Input: part model. Units: mm. Frame: model coordinates. A direction names the side the tool comes from. Give positions to 0.01 mm unless a question says otherwise; leave off trailing zeros. Loops run counter-clockwise (first coordinate to the right, second up) from the corner with the lowest first, then second, coordinate; pieces in that order, holes last. Notation, with made-up numbers: (2.25, -33.75) - (17.25, -33.75) arc R17 ccw to (17.25, -14.75) - close; hole circle Ø10 at (69.5, 54). An arc over 180 degrees is marked (long way). Answer as a JSON object with one key per item and string values. Group by question number.
(1) Pin query (flat end, axial travel): P1, Ø10, axis at y = 1.5, z = 12, coming from the -X side; P2, Ø2, axis at y = 26, z = 8, coming from the +X side; P3, Ø3, axis at x = 11, y = 24.5, coming from the -Z side. Return the tip coordinate at first contact, or that it passes through.
(2) Section query B-B (z = 11.5). Return loops of the section in (x, y), plus the area to 3 significant figures.
(3) Mould query, pull axis X, two halves, no side actions, for faces 4 (the flat face through (3.127, -26.5, 11.3)), 5 (the flat face through (16, 0, 11)), 6 (the flat face through (6, -17.5, 11)). Classes: +X half, -X half, draft (parallel to the pull), parting line (faces both ways), or undercut.
(4) Section query A-A (x = 8.75). Return loops of the section in (y, z).
(5) Section query C-C (y = -23.4). Return loops of the section in (x, z), plus the area to 3 significant figures.
(6) Access query for faces 1 (the flat face through (13, 0, 11)), 2 (the flat face through (9, -23, 14.75)), 3 (the flat face through (8, 24, 14.75)). Directions: +Z, -Z, +X, -X, +Y, -Y. A direction counts if a zero-diameter tool reaches every point of the face in a straight line with its end or side. Return the directions, or none.
(7) Section query D-D (x = 12). Return loops of the section in (y, z), plus the area to 3 significant figures.
(8) Material intervals for L1, parallel to Y at x = 6.5, z = 3.75; L2, parallel to Z at x = 1.8, y = -24.25; L3, parallel to Y at x = 12.75, z = 15, sorted ascending.
```python
from build123d import *

# Parameters (mm, degrees)
BOSS_EXTRUDE1_DEPTH = 23
SKETCH2_R           = 1.7
CUT_EXTRUDE1_DEPTH  = 39.81958977
CUT_EXTRUDE5_START  = 23
SKETCH2_8_R         = 3.25
SKETCH2_8_R_2       = 1.7
CUT_EXTRUDE5_DEPTH  = 23
MIRROR5_START       = 14.75
MIRROR5_OUTLINE_W   = 3.127139018
MIRROR5_OUTLINE_H   = 0.5
MIRROR5_DEPTH       = 8.25
MIRROR5_2_OUTLINE_W = 3.127139018
MIRROR5_2_OUTLINE_H = 0.5
MIRROR5_2_DEPTH     = 14.75
MIRROR5_3_OUTLINE_W = 13
MIRROR5_3_OUTLINE_H = 0.5
MIRROR5_3_DEPTH     = 23
MIRROR5_4_OUTLINE_R = 1.7
MIRROR5_4_DEPTH     = 3.127139018
MIRROR5_5_OUTLINE_R = 1.7
MIRROR5_5_DEPTH     = 3.127139018
SKETCH5_R           = 1.7
CUT_EXTRUDE6_DEPTH  = 41.323690307
CUT_EXTRUDE7_DEPTH  = 23


with BuildPart() as part:
    # Sketch1 → Boss-Extrude1 (new body)
    with BuildSketch(Plane.XY):
        with BuildLine():
            Line((13, 18), (13, -18))
            Line((13, -18), (0, -18))
            Line((0, -18), (0, -28.5))
            Line((0, -28.5), (3.127139018, -28.5))
            Line((3.127139018, -28.5), (3.127139018, -21))
            Line((3.127139018, -21), (16, -21))
            Line((16, -21), (16, 21))
            ThreePointArc((16, 21), (9.563569509, 27.436430491), (3.127139018, 21))
            Line((3.127139018, 21), (3.127139018, 28.5))
            Line((3.127139018, 28.5), (0, 28.5))
            Line((0, 28.5), (0, 18))
            Line((0, 18), (13, 18))
        make_face()
    extrude(amount=BOSS_EXTRUDE1_DEPTH)

    # Sketch2 → Cut-Extrude1 (cut, symmetric)
    with BuildSketch(Plane(origin=(3.127139018, 0, 0), x_dir=(0, 0, -1), z_dir=(1, 0, 0))):
        with Locations((-11.5, 24.75)):
            Circle(SKETCH2_R)
    extrude(amount=CUT_EXTRUDE1_DEPTH, both=True, mode=Mode.SUBTRACT)

    # Sketch2_8 → Cut-Extrude5 (cut)
    # profile 1 of 4: a face of its own
    with BuildSketch(Plane(origin=(3.127139018, 0, 0), x_dir=(0, 0, -1), z_dir=(1, 0, 0)).offset(CUT_EXTRUDE5_START)):
        with BuildLine():
            Line((-14.75, 28.5), (-14.75, 24.75))
            ThreePointArc((-14.75, 24.75), (-11.5, 28), (-8.25, 24.75))
            Line((-8.25, 24.75), (-8.25, 28.5))
            Line((-8.25, 28.5), (-14.75, 28.5))
        make_face()
    # profile 2 of 4: a face of its own
    with BuildSketch(Plane(origin=(3.127139018, 0, 0), x_dir=(0, 0, -1), z_dir=(1, 0, 0)).offset(CUT_EXTRUDE5_START)):
        with Locations((-11.5, 24.75)):
            Circle(SKETCH2_8_R)
        with Locations((-11.5, 24.75)):
            Circle(SKETCH2_8_R_2, mode=Mode.SUBTRACT)
    # profile 3 of 4: a face of its own
    with BuildSketch(Plane(origin=(3.127139018, 0, 0), x_dir=(0, 0, -1), z_dir=(1, 0, 0)).offset(CUT_EXTRUDE5_START)):
        with BuildLine():
            ThreePointArc((-11.5, 21.5), (-13.798097039, 22.451902961), (-14.75, 24.75))
            Line((-14.75, 24.75), (-14.75, 21.5))
            Line((-14.75, 21.5), (-11.5, 21.5))
        make_face()
    # profile 4 of 4: a face of its own
    with BuildSketch(Plane(origin=(3.127139018, 0, 0), x_dir=(0, 0, -1), z_dir=(1, 0, 0)).offset(CUT_EXTRUDE5_START)):
        with BuildLine():
            Line((-8.25, 28.5), (-8.25, 24.75))
            ThreePointArc((-8.25, 24.75), (-9.201902961, 22.451902961), (-11.5, 21.5))
            Line((-11.5, 21.5), (0, 21.5))
            Line((0, 21.5), (0, 28.5))
            Line((0, 28.5), (-8.25, 28.5))
        make_face()
    extrude(amount=-CUT_EXTRUDE5_DEPTH, mode=Mode.SUBTRACT)

    # Mirror5: read off the stored shape, not the designer's step
    # Mirror5 outline → Mirror5 (add)
    with BuildSketch(Plane.XY.offset(MIRROR5_START)):
        with BuildLine():
            ThreePointArc((3.146589108, -21), (9.563569509, -26.936430491), (15.98054991, -21))
            Line((15.98054991, -21), (3.146589108, -21))
        make_face()
        with Locations((1.563569509, 28.75)):
            Rectangle(MIRROR5_OUTLINE_W, MIRROR5_OUTLINE_H)
    extrude(amount=MIRROR5_DEPTH)

    # Mirror5 2 outline → Mirror5 2 (add)
    with BuildSketch(Plane.XY):
        with Locations((1.563569509, 28.75)):
            Rectangle(MIRROR5_2_OUTLINE_W, MIRROR5_2_OUTLINE_H)
    extrude(amount=MIRROR5_2_DEPTH)

    # Mirror5 3 outline → Mirror5 3 (add)
    with BuildSketch(Plane.XY):
        with Locations((6.5, -17.75)):
            Rectangle(MIRROR5_3_OUTLINE_W, MIRROR5_3_OUTLINE_H)
        with BuildLine():
            ThreePointArc((3.127139018, 21), (3.132003379, 21.250189081), (3.146589108, 21.5))
            Line((3.146589108, 21.5), (3.127139018, 21.5))
            Line((3.127139018, 21.5), (3.127139018, 21))
        make_face()
        with BuildLine():
            Line((16, 21), (16, 21.5))
            Line((16, 21.5), (15.98054991, 21.5))
            ThreePointArc((15.98054991, 21.5), (15.995135639, 21.250189081), (16, 21))
        make_face()
    extrude(amount=MIRROR5_3_DEPTH)

    # Mirror5 4 outline → Mirror5 4 (cut)
    with BuildSketch(Plane.YZ):
        with Locations((-24.25, 11.5)):
            Circle(MIRROR5_4_OUTLINE_R)
    extrude(amount=MIRROR5_4_DEPTH, mode=Mode.SUBTRACT)

    # Mirror5 5 outline → Mirror5 5 (add)
    with BuildSketch(Plane.YZ):
        with Locations((24.75, 11.5)):
            Circle(MIRROR5_5_OUTLINE_R)
    extrude(amount=MIRROR5_5_DEPTH)

    # Sketch5 → Cut-Extrude6 (cut, through all)
    with BuildSketch(Plane.XY.offset(23)):
        with Locations((11.2, 23.9)):
            Circle(SKETCH5_R)
    cut_extrude6 = extrude(amount=-CUT_EXTRUDE6_DEPTH, mode=Mode.SUBTRACT)

    # Mirror8: Cut-Extrude6 across plane
    add(cut_extrude6.mirror(Plane(origin=(0, 0.25, 0), x_dir=(0, 0, 1), z_dir=(0, -1, 0))), mode=Mode.SUBTRACT)

    # Sketch6 → Cut-Extrude7 (cut)
    with BuildSketch(Plane(origin=(3.127139018, 0, 0), x_dir=(0, 0, -1), z_dir=(1, 0, 0))):
        with BuildLine():
            ThreePointArc((-9.883759273, 25.77703502), (-11.5, 26.95), (-13.116240727, 25.77703502))
            Line((-13.116240727, 25.77703502), (-11.5, 25.25))
            Line((-11.5, 25.25), (-9.883759273, 25.77703502))
        make_face()
        with BuildLine():
            Line((-11.5, 25.25), (-13.116240727, 25.77703502))
            ThreePointArc((-13.116240727, 25.77703502), (-13.2, 25.25), (-13.116240727, 24.72296498))
            Line((-13.116240727, 24.72296498), (-11.5, 25.25))
        make_face()
        with BuildLine():
            Line((-9.883759273, 25.77703502), (-11.5, 25.25))
            Line((-11.5, 25.25), (-9.883759273, 24.72296498))
            ThreePointArc((-9.883759273, 24.72296498), (-9.821070395, 24.983175372), (-9.8, 25.25))
            ThreePointArc((-9.8, 25.25), (-9.821070395, 25.516824628), (-9.883759273, 25.77703502))
        make_face()
        with BuildLine():
            Line((-9.883759273, 24.72296498), (-11.5, 25.25))
            Line((-11.5, 25.25), (-13.116240727, 24.72296498))
            ThreePointArc((-13.116240727, 24.72296498), (-11.5, 23.55), (-9.883759273, 24.72296498))
        make_face()
    extrude(amount=-CUT_EXTRUDE7_DEPTH, mode=Mode.SUBTRACT)


solid = part.part
```
Recorded:
{
 "1": {"P1": "stops at x = 13", "P2": "stops at x = 3.13", "P3": "stops at z = 14.75"},
 "2": {"outline": "(0, -28.5) - (3.13, -28.5) - (3.13, -25.95) - (0, -25.95) - close; (0, -22.55) - (3.13, -22.55) - (3.13, -21) - (16, -21) - (16, 21.5) - (3.13, 21.5) - (3.13, 23.55) - (0, 23.55) - (0, 18) - (13, 18) - (13, -17.5) - (0, -17.5) - close; (0, 26.95) - (3.13, 26.95) - (3.13, 29) - (0, 29) - close", "area": "244 mm^2"},
 "3": {"face 4": "undercut", "face 5": "+X half", "face 6": "draft"},
 "4": {"outline": "(-26.88, 14.75) - (-21, 14.75) - (-21, 0) - (-17.5, 0) - (-17.5, 23) - (-26.88, 23) - close; (18, 0) - (21.5, 0) - (21.5, 14.75) - (27.38, 14.75) - (27.38, 23) - (18, 23) - close"},
 "5": {"outline": "(0, 0) - (3.13, 0) - (3.13, 10.03) - (0, 10.03) - close; (0, 12.97) - (3.13, 12.97) - (3.13, 23) - (0, 23) - close; (3.82, 14.75) - (9.5, 14.75) - (9.5, 23) - (3.82, 23) - close; (12.9, 14.75) - (15.31, 14.75) - (15.31, 23) - (12.9, 23) - close", "area": "129 mm^2"},
 "6": {"face 1": "+Z, -Z, -X", "face 2": "-Z, +X, -Y", "face 3": "-Z, +X, +Y"},
 "7": {"outline": "(-26.46, 14.75) - (-24.9, 14.75) - (-24.9, 23) - (-26.46, 23) - close; (-21.9, 14.75) - (-21, 14.75) - (-21, 0) - (-17.5, 0) - (-17.5, 23) - (-21.9, 23) - close; (18, 0) - (21.5, 0) - (21.5, 14.75) - (22.4, 14.75) - (22.4, 23) - (18, 23) - close; (25.4, 14.75) - (26.96, 14.75) - (26.96, 23) - (25.4, 23) - close", "area": "202 mm^2"},
 "8": {"L1": "y = -21 to -17.5, 18 to 21.5", "L2": "z = 0 to 9.8, 13.2 to 23", "L3": "y = -26.09 to -24.1, -22.7 to -17.5, 18 to 23.2, 24.6 to 26.59"}
}
